```python
from build123d import *

# Parameters (mm, degrees)
SKETCH1_R               = 1.5
SKETCH1_R_2             = 18.5
SKETCH1_R_3             = 17.5
BOSS_EXTRUDE1_DEPTH     = 1.5
SKETCH1_4_R             = 18.5
SKETCH1_4_R_2           = 17.5
BOSS_EXTRUDE2_DEPTH     = 61.5
CUT_EXTRUDE1_START      = -61.5
SKETCH1_5_R             = 17.5
CUT_EXTRUDE1_DEPTH      = 6
SKETCH2_R               = 9.5
SKETCH2_R_2             = 5.75
BOSS_EXTRUDE3_DEPTH     = 8.5
SKETCH3_R               = 5.75
CUT_EXTRUDE2_DEPTH      = 1
SKETCH4_R               = 3
CUT_EXTRUDE3_DEPTH      = 79.183366667
CUT_EXTRUDE3_DEPTH_BACK = 79.183366667
CUT_EXTRUDE4_START      = -1.5
SKETCH5_R               = 18.5
SKETCH5_R_2             = 17.5
CUT_EXTRUDE4_DEPTH      = 0.25
SKETCH6_R               = 18.5
CUT_EXTRUDE5_DEPTH      = 0.5


with BuildPart() as part:
    # Sketch1 → Boss-Extrude1 (new body)
    with BuildSketch(Plane(origin=(0, 0, 0), x_dir=(0, 0, -1), z_dir=(1, 0, 0))):
        with BuildLine():
            ThreePointArc((-11.366411782, 18.755724012), (-16.300215512, 19.152688435), (-16.697179934, 14.218884704))
            Line((-16.697179934, 14.218884704), (-14.710366227, 11.218517079))
            ThreePointArc((-14.710366227, 11.218517079), (-11.99021817, 14.088458689), (-8.722294226, 16.31476581))
            Line((-8.722294226, 16.31476581), (-11.366411782, 18.755724012))
        make_face()
        with Locations((-14.031795858, 16.487304358)):
            Circle(SKETCH1_R, mode=Mode.SUBTRACT)
        Circle(SKETCH1_R_2)
        Circle(SKETCH1_R_3, mode=Mode.SUBTRACT)
        Circle(SKETCH1_R_3)
        with BuildLine():
            Line((17.42629206, 13.315286142), (14.061297684, 12.022059201))
            ThreePointArc((14.061297684, 12.022059201), (16.304113863, 8.74218915), (17.794831776, 5.059047546))
            Line((17.794831776, 5.059047546), (20.734147414, 7.146161977))
            ThreePointArc((20.734147414, 7.146161977), (22.164781819, 11.884651736), (17.42629206, 13.315286142))
        make_face()
        with Locations((19.080219737, 10.230724059)):
            Circle(SKETCH1_R, mode=Mode.SUBTRACT)
        with BuildLine():
            ThreePointArc((3.927811116, -18.078227232), (0, -18.5), (-3.927811116, -18.078227232))
            Line((-3.927811116, -18.078227232), (-3.5, -21.65))
            ThreePointArc((-3.5, -21.65), (0, -25.15), (3.5, -21.65))
            Line((3.5, -21.65), (3.927811116, -18.078227232))
        make_face()
        with Locations((0, -21.65)):
            Circle(SKETCH1_R, mode=Mode.SUBTRACT)
    extrude(amount=BOSS_EXTRUDE1_DEPTH)

    # Sketch1<4> → Boss-Extrude2 (add)
    with BuildSketch(Plane(origin=(0, 0, 0), x_dir=(0, 0, -1), z_dir=(1, 0, 0))):
        with Locations(Location((0, 0, 0), (0, 0, 142.669891736))):
            Circle(SKETCH1_4_R)
        Circle(SKETCH1_4_R_2, mode=Mode.SUBTRACT)
        Circle(SKETCH1_4_R_2)
    extrude(amount=-BOSS_EXTRUDE2_DEPTH)

    # Sketch1<5> → Cut-Extrude1 (cut)
    with BuildSketch(Plane(origin=(0, 0, 0), x_dir=(0, 0, -1), z_dir=(1, 0, 0)).offset(CUT_EXTRUDE1_START)):
        Circle(SKETCH1_5_R)
    extrude(amount=CUT_EXTRUDE1_DEPTH, mode=Mode.SUBTRACT)

    # Sketch2 → Boss-Extrude3 (add)
    with BuildSketch(Plane(origin=(1.5, 0, 0), x_dir=(0, 0, -1), z_dir=(1, 0, 0))):
        Circle(SKETCH2_R)
        Circle(SKETCH2_R_2, mode=Mode.SUBTRACT)
        Circle(SKETCH2_R_2)
    extrude(amount=BOSS_EXTRUDE3_DEPTH)

    # Sketch3 → Cut-Extrude2 (cut)
    with BuildSketch(Plane(origin=(10, 0, 0), x_dir=(0, 0, -1), z_dir=(1, 0, 0))):
        Circle(SKETCH3_R)
    extrude(amount=-CUT_EXTRUDE2_DEPTH, mode=Mode.SUBTRACT)

    # Sketch4 → Cut-Extrude3 (cut, two sides)
    with BuildSketch(Plane(origin=(9, 0, 0), x_dir=(0, 0, -1), z_dir=(1, 0, 0))) as cut_extrude3_sk:
        Circle(SKETCH4_R)
    extrude(amount=CUT_EXTRUDE3_DEPTH, mode=Mode.SUBTRACT)
    extrude(cut_extrude3_sk.sketch, amount=-CUT_EXTRUDE3_DEPTH_BACK, mode=Mode.SUBTRACT)

    # Sketch5 → Cut-Extrude4 (cut)
    with BuildSketch(Plane(origin=(1.5, 0, 0), x_dir=(0, 0, -1), z_dir=(1, 0, 0)).offset(CUT_EXTRUDE4_START)):
        Circle(SKETCH5_R)
        Circle(SKETCH5_R_2, mode=Mode.SUBTRACT)
    extrude(amount=-CUT_EXTRUDE4_DEPTH, mode=Mode.SUBTRACT)

    # Sketch6 → Cut-Extrude5 (cut)
    with BuildSketch(Plane.ZY.offset(61.5)):
        Circle(SKETCH6_R)
    extrude(amount=-CUT_EXTRUDE5_DEPTH, mode=Mode.SUBTRACT)


solid = part.part
```
Geometry check sheet. Reference: the model listing, model coordinates, mm. A direction names the side the tool comes from. Round coordinates to 2 decimals unless told otherwise and drop trailing zeros. Loops run counter-clockwise (first coordinate to the right, second up) from the corner with the lowest first, then second, coordinate; pieces in that order, holes last. Notation, with made-up numbers: (71.25, 31.25) -> (97.25, 31.25) arc R13 cw to (97.25, 54.25) -> close; hole circle Ø5 at (83.5, -12.5). An arc over 180 degrees is marked (long way). Use a Markdown table: item, result.
(1) Scan lines: probe 1 along Y at (x, z) = (-11.5, 0); probe 2 along Y at (x, z) = (-59.7, 0); probe 3 along X at (y, z) = (-18, -0.5). Record each from-to range of solid material in increasing order.
Calculated:
| item | result |
|---|---|
| probe 1 | -18.5 to -3, 3 to 18.5 |
| probe 2 | -18.5 to -17.5, 17.5 to 18.5 |
| probe 3 | -61 to -0.25, 0 to 1.5 |
(2) Sectioned sample at D-D (z = -8). Enter the section's corners in (x, y), then the cut area to 3 significant figures.
Calculated:
| item | result |
|---|---|
| outline | (-61, -16.68) -> (-0.25, -16.68) -> (-0.25, -15.56) -> (0, -15.56) -> (0, -16.68) -> (1.5, -16.68) -> (1.5, -5.12) -> (10, -5.12) -> (10, 5.12) -> (1.5, 5.12) -> (1.5, 16.68) -> (0, 16.68) -> (0, 15.56) -> (-0.25, 15.56) -> (-0.25, 16.68) -> (-61, 16.68) -> (-61, 15.56) -> (-55.5, 15.56) -> (-55.5, -15.56) -> (-61, -15.56) -> close |
| area | 2,000 mm² |
(3) Go/stop test with flat-tipped pins: P1, Ø12.5, axis at y = -4.5, z = -7, coming from the -X side; P2, Ø1, axis at x = 0, y = 5, coming from the +Z side; P3, Ø5, axis at x = -43.5, z = 11.5, coming from the -Y side. Record where each tip stops, or that it passes through.
Calculated:
| item | result |
|---|---|
| P1 | x = -55.5 |
| P2 | z = 17.94 |
| P3 | y = -16.16 |
(4) Mould release check, pull along X, two halves, no side actions. Record for faces 1 (the flat face through (0, 18, 0)), 2 (the flat face through (1.5, 8, -6)), 3 (the flat face through (-55.5, -4, 0)): released by +X, released by -X, zero draft, split by the parting line, or undercut.
Calculated:
| item | result |
|---|---|
| face 1 | undercut |
| face 2 | released by +X |
| face 3 | released by -X |
(5) Set-up check for faces 4 (the cylindrical face through (-58.288, -10.648, 13.887)), 5 (the flat face through (0.74, -19.839, 3.717)), 6 (the flat face through (0.74, 12.68, -15.77)), 7 (the flat face through (0.74, 6.088, -19.244)), 8 (the cylindrical face through (0.74, -20.163, 0.195)): record each of +Z, -Z, +X, -X, +Y, -Y from which the full face is reachable in a straight line by a thin tool's end or side.
Calculated:
| item | result |
|---|---|
| face 4 | -X |
| face 5 | +Z, +X, -X, -Y |
| face 6 | +X, -X, +Y |
| face 7 | -Z, +X, -X |
| face 8 | +X, -X |
(6) Sectioned sample at B-B (y = 0). Enter the section's corners in (x, z), then the cut area to 3 significant figures.
Calculated:
| item | result |
|---|---|
| outline | (-61, -18.5) -> (-0.25, -18.5) -> (-0.25, -17.5) -> (0, -17.5) -> (0, -18.5) -> (1.5, -18.5) -> (1.5, -9.5) -> (10, -9.5) -> (10, -5.75) -> (9, -5.75) -> (9, -3) -> (-55.5, -3) -> (-55.5, -17.5) -> (-61, -17.5) -> close; (-61, 17.5) -> (-55.5, 17.5) -> (-55.5, 3) -> (9, 3) -> (9, 5.75) -> (10, 5.75) -> (10, 9.5) -> (1.5, 9.5) -> (1.5, 18.5) -> (0, 18.5) -> (0, 17.5) -> (-0.25, 17.5) -> (-0.25, 18.5) -> (-61, 18.5) -> close |
| area | 1,880 mm² |
(7) Sectioned sample at C-C (x = 5.5). Enter the section's corners in (y, z).
Calculated:
| item | result |
|---|---|
| outline | circle Ø19 at (0, 0); hole circle Ø6 at (0, 0) |
(8) Sectioned sample at A-A (z = 0). Give the number of separate pieces and of enclosed holes in the cut face, then the cut area to 3 significant figures.
Calculated:
| item | result |
|---|---|
| separate pieces | 3 |
| enclosed holes | 0 |
| area | 1,890 mm² |
